Input: part model. Units: mm. Frame: model coordinates. Face numbers are marked on the shaded views. A direction names the side the tool comes from. Coordinates: 2 decimals unless noted, no trailing zeros. Order: outer loops, then holes, each group sorted by start corner. A loop starts at its lowest first (then second) coordinate and runs counter-clockwise, first axis right, second up. Notation, with made-up numbers: (41, -23) -> (54, -23) arc R22 cw to (54, 8) -> close; hole circle Ø3 at (85, 5). An arc over 180 degrees is marked (long way). Answer as CSV lines item,"result".
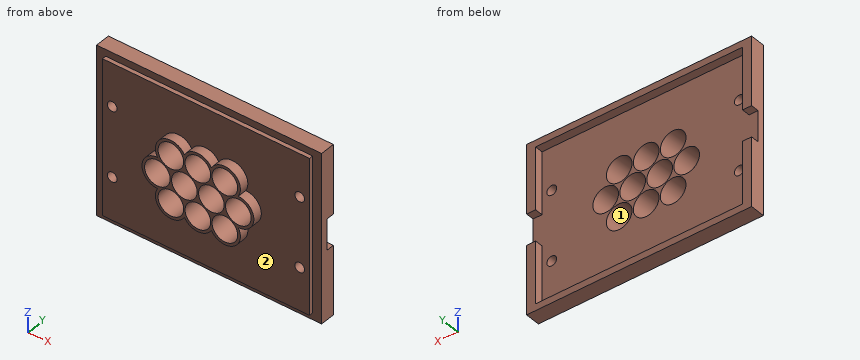
Autodesk Inventor part; units mm, degrees
ref_plane "YZ Plane" through (0, 0, 0) normal (1, 0, 0) x (0, 1, 0)
ref_plane "XZ Plane" through (0, 0, 0) normal (0, 1, 0) x (-1, 0, 0)
ref_plane "XY Plane" through (0, 0, 0) normal (0, 0, 1) x (1, 0, 0)
sketch "Sketch1" plane through (0, 0, 0) normal (0, 1, 0) x (-1, 0, 0)
  circle A0 centre (0, 0) radius 9.5
  circle A1 centre (20, 0) radius 9.5
  circle A2 centre (-20, 0) radius 9.5
  circle A3 centre (-10, 17.3205) radius 9.5
  circle A4 centre (10, 17.3205) radius 9.5
  circle A5 centre (30, 17.3205) radius 9.5
  circle A6 centre (10, -17.3205) radius 9.5
  circle A7 centre (30, -17.3205) radius 9.5
  circle A8 centre (-10, -17.3205) radius 9.5
  circle A9 centre (40, 0) radius 9.5
  line L0 (0, 0) -> (-32.9562, 0) construction
  line L1 (-32.9562, 0) -> (61.076, 0) construction
  circle A10 centre (0, 0) radius 10.5 construction
  circle A11 centre (-20, 0) radius 10.5 construction
  circle A12 centre (-10, -17.3205) radius 10.5 construction
  circle A13 centre (10, -17.3205) radius 10.5 construction
  circle A14 centre (30, -17.3205) radius 10.5 construction
  circle A15 centre (40, 0) radius 10.5 construction
  circle A16 centre (20, 0) radius 10.5 construction
  circle A17 centre (30, 17.3205) radius 10.5 construction
  circle A18 centre (10, 17.3205) radius 10.5 construction
  circle A19 centre (-10, 17.3205) radius 10.5 construction
  circle A20 centre (40, 0) radius 11.5 construction
  circle A21 centre (30, -17.3205) radius 11.5 construction
  circle A22 centre (10, -17.3205) radius 11.5 construction
  circle A23 centre (-10, -17.3205) radius 11.5 construction
  circle A24 centre (-20, 0) radius 11.5 construction
  circle A25 centre (-10, 17.3205) radius 11.5 construction
  circle A26 centre (10, 17.3205) radius 11.5 construction
  circle A27 centre (30, 17.3205) radius 11.5 construction
  circle A28 centre (0, 0) radius 11.5 construction
  circle A29 centre (20, 0) radius 11.5 construction
  arc A30 (39.9181, -11.4997) -> (39.9181, 11.4997) centre (39.9181, 0) ccw
  arc A31 (39.9181, 11.4997) -> (20, 22.9994) centre (30, 17.3205) ccw
  arc A32 (20, 22.9994) -> (0, 22.9994) centre (10, 17.3205) ccw
  arc A33 (0, 22.9994) -> (-19.9181, 11.4997) centre (-10, 17.3205) ccw
  arc A34 (-19.9181, 11.4997) -> (-19.9181, -11.4997) centre (-20, 0) ccw
  arc A35 (-19.9181, -11.4997) -> (0, -22.9994) centre (-10, -17.3205) ccw
  arc A36 (0, -22.9994) -> (20, -22.9994) centre (10, -17.3205) ccw
  arc A37 (20, -22.9994) -> (39.9181, -11.4997) centre (30, -17.3205) ccw
  point P0 (28.893, 7.4235)
  dimension "d0" = 19
  dimension "d2" = 19
  dimension "d4" = 19
  dimension "d6" = 19
  dimension "d8" = 19
  dimension "d10" = 19
  dimension "d11" = 19
  dimension "d13" = 19
  dimension "d14" = 19
  dimension "d53" = 19
  dimension "d91" = 1
  dimension "d144" = 21
  dimension "d145" = 21
  dimension "d146" = 21
  dimension "d147" = 21
  dimension "d148" = 21
  dimension "d149" = 21
  dimension "d150" = 21
  dimension "d151" = 21
  dimension "d152" = 21
  dimension "d153" = 21
  dimension "d154" = 23
  dimension "d155" = 23
  dimension "d156" = 23
  dimension "d157" = 23
  dimension "d158" = 23
  dimension "d159" = 23
  dimension "d160" = 23
  dimension "d161" = 23
  dimension "d162" = 23
  dimension "d163" = 23
extrude "Extrusion1" add sketch "Sketch1" along normal blind 15
sketch "Sketch4" plane through (0, 15, 0) normal (0, 1, 0) x (1, 0, 0)
  circle A0 centre (-30, 17.3205) radius 9.5
  circle A1 centre (-40, 0) radius 9.5
  circle A2 centre (-40, 0) radius 9.5
  circle A3 centre (10, 17.3205) radius 9.5
  circle A4 centre (-30, 17.3205) radius 9.5
  circle A5 centre (-10, 17.3205) radius 9.5
  circle A6 centre (-30, -17.3205) radius 9.5
  circle A7 centre (-10, -17.3205) radius 9.5
  circle A8 centre (10, -17.3205) radius 9.5
  circle A9 centre (20, 0) radius 9.5
  circle A10 centre (-20, 0) radius 9.5
  circle A11 centre (0, 0) radius 9.5
  line L0 (0, 0) -> (-9.528, 0) construction
  line L1 (-86.228, 57.7) -> (67.172, 57.7)
  line L2 (67.172, 57.7) -> (67.172, -57.7)
  line L3 (67.172, -57.7) -> (-86.228, -57.7)
  line L4 (-86.228, -57.7) -> (-86.228, 57.7)
  line L5 (-86.228, 57.7) -> (67.172, -57.7) construction
  line L6 (67.172, 57.7) -> (-86.228, -57.7) construction
  arc A12 (0, 22.9994) -> (-20, 22.9994) centre (-10, 17.3205) ccw
  arc A13 (19.9181, 11.4997) -> (0, 22.9994) centre (10, 17.3205) ccw
  arc A14 (19.9181, -11.4997) -> (19.9181, 11.4997) centre (20, 0) ccw
  arc A15 (0, -22.9994) -> (19.9181, -11.4997) centre (10, -17.3205) ccw
  arc A16 (-20, -22.9994) -> (0, -22.9994) centre (-10, -17.3205) ccw
  arc A17 (-39.9181, -11.4997) -> (-20, -22.9994) centre (-30, -17.3205) ccw
  circle A18 centre (-30, 17.3205) radius 11.5 construction
  arc A19 (-39.9181, 11.4997) -> (-39.9181, -11.4997) centre (-39.9181, 0) ccw
  arc A20 (-20, 22.9994) -> (-39.9181, 11.4997) centre (-30, 17.3205) ccw
  arc A21 (0, 22.9994) -> (-20, 22.9994) centre (-10, 17.3205) ccw
  arc A22 (19.9181, 11.4997) -> (0, 22.9994) centre (10, 17.3205) ccw
  arc A23 (19.9181, -11.4997) -> (19.9181, 11.4997) centre (20, 0) ccw
  arc A24 (0, -22.9994) -> (19.9181, -11.4997) centre (10, -17.3205) ccw
  arc A25 (-20, -22.9994) -> (0, -22.9994) centre (-10, -17.3205) ccw
  arc A26 (-39.9181, -11.4997) -> (-20, -22.9994) centre (-30, -17.3205) ccw
  arc A27 (-39.9181, 11.4997) -> (-39.9181, -11.4997) centre (-39.9181, 0) ccw
  arc A28 (-20, 22.9994) -> (-39.9181, 11.4997) centre (-30, 17.3205) ccw
  point P0 (-17.0502, -21.4927)
  point P1 (-17.0502, -11.5134)
  point P2 (-17.0502, -8.8009)
  point P3 (-17.0502, 8.8009)
  point P4 (-17.0502, 11.5134)
  point P5 (-17.0502, 21.4927)
  point P6 (-2.0059, 21.4927)
  point P7 (-2.0059, -11.5134)
  point P8 (-2.0059, -8.8009)
  point P9 (-2.0059, 8.8009)
  point P10 (-2.0059, 11.5134)
  point P11 (-2.0059, -21.4927)
  dimension "d104" = 153.4
  dimension "d164" = 115.4
extrude "Extrusion7" add sketch "Sketch4" against normal blind 8 contours L1 L2 L3 L4
sketch "Sketch5" plane through (0, 15, 0) normal (0, 1, 0) x (1, 0, 0)
  line L0 (-86.228, -57.7) -> (67.172, -57.7)
  line L1 (67.172, -57.7) -> (67.172, 57.7)
  line L2 (67.172, 57.7) -> (-86.228, 57.7)
  line L3 (-86.228, 57.7) -> (-86.228, -57.7)
  circle A0 centre (-40, 0) radius 9.5
  circle A1 centre (10, 17.3205) radius 9.5
  circle A2 centre (-30, 17.3205) radius 9.5
  circle A3 centre (-10, 17.3205) radius 9.5
  circle A4 centre (-30, -17.3205) radius 9.5
  circle A5 centre (-10, -17.3205) radius 9.5
  circle A6 centre (10, -17.3205) radius 9.5
  circle A7 centre (20, 0) radius 9.5
  circle A8 centre (-20, 0) radius 9.5
  circle A9 centre (0, 0) radius 9.5
  line L4 (-86.228, 57.7) -> (67.172, 57.7)
  line L5 (67.172, 57.7) -> (67.172, -57.7)
  line L6 (67.172, -57.7) -> (-86.228, -57.7)
  line L7 (-86.228, -57.7) -> (-86.228, 57.7)
  line L8 (-92.8745, -62.7) -> (73.8184, -62.7)
  line L9 (73.8184, -62.7) -> (73.8184, 62.7)
  line L10 (73.8184, 62.7) -> (-92.8745, 62.7)
  line L11 (-92.8745, 62.7) -> (-92.8745, -62.7)
  line L12 (-92.8745, -62.7) -> (73.8184, 62.7) construction
  line L13 (73.8184, -62.7) -> (-92.8745, 62.7) construction
  point P0 (66.922, -57.45)
  point P1 (-9.528, 0)
  dimension "d169" = 5
  dimension "d170" = 6.6464
  dimension "d171" = 166.6929
  dimension "d172" = 125.4
extrude "Extrusion8" add sketch "Sketch5" along normal blind 6 and the other way blind 5 contours L11 L10 L9 L8
sketch "Sketch6" plane through (0, 15, 0) normal (0, 1, 0) x (1, 0, 0)
  line L0 (59.944, 57.1514) -> (59.944, 25.95) construction
  line L1 (59.944, 25.95) -> (67.172, 25.95) construction
  line L2 (-79, -57.7) -> (-79, -25.95) construction
  line L3 (-79, -25.95) -> (-86.228, -25.95) construction
  circle A0 centre (59.944, 25.95) radius 3.615
  circle A1 centre (59.944, -25.95) radius 3.615
  circle A2 centre (-79, -25.95) radius 3.615
  circle A3 centre (-79, 25.95) radius 3.615
  line L4 (73.8184, -62.7) -> (73.8184, 62.7)
  line L5 (73.8184, 62.7) -> (-92.8745, 62.7)
  line L6 (-92.8745, 62.7) -> (-92.8745, -62.7)
  line L7 (-92.8745, -62.7) -> (73.8184, -62.7)
  line L8 (-86.228, -57.7) -> (-86.228, 57.7)
  line L9 (-86.228, 57.7) -> (67.172, 57.7)
  line L10 (67.172, 57.7) -> (67.172, -57.7)
  line L11 (67.172, -57.7) -> (-86.228, -57.7)
  line L12 (-86.228, -57.7) -> (67.172, -57.7)
  line L13 (67.172, -57.7) -> (67.172, 57.7)
  line L14 (67.172, 57.7) -> (-86.228, 57.7)
  line L15 (-86.228, 57.7) -> (-86.228, -57.7)
  circle A4 centre (-40, 0) radius 9.5
  circle A5 centre (10, 17.3205) radius 9.5
  circle A6 centre (-30, 17.3205) radius 9.5
  circle A7 centre (-10, 17.3205) radius 9.5
  circle A8 centre (-30, -17.3205) radius 9.5
  circle A9 centre (-10, -17.3205) radius 9.5
  circle A10 centre (10, -17.3205) radius 9.5
  circle A11 centre (20, 0) radius 9.5
  circle A12 centre (-20, 0) radius 9.5
  circle A13 centre (0, 0) radius 9.5
  line L16 (-86.228, 57.7) -> (67.172, 57.7)
  line L17 (67.172, 57.7) -> (67.172, -57.7)
  line L18 (67.172, -57.7) -> (-86.228, -57.7)
  line L19 (-86.228, -57.7) -> (-86.228, 57.7)
  dimension "d123" = 7.23
  dimension "d124" = 7.23
  dimension "d125" = 7.23
  dimension "d140" = 7.23
  dimension "d179" = 31.75
  dimension "d180" = 7.228
  dimension "d181" = 7.228
  dimension "d182" = 31.75
  dimension "d183" = 31.75
  dimension "d184" = 7.228
  dimension "d185" = 7.228
  dimension "d186" = 31.75
extrude "Extrusion6" cut sketch "Sketch6" against normal through all contours A0 | A1 | A2 | A3
sketch "Sketch7" plane through (-92.8745, 10, 62.7) normal (-1, 0, 0) x (0, 0, 1)
  line L0 (-74.1997, -10) -> (-74.1997, -3)
  line L1 (-51.2003, -10) -> (-51.2003, -3)
  line L2 (-120.4, 5) -> (-5, 5)
  line L3 (0, 0) -> (-125.4, 0)
  line L4 (-125.4, 11) -> (0, 11)
  line L5 (-74.1997, 5) -> (-51.2003, 5)
  line L6 (-51.2003, 5) -> (-51.2003, 11)
  line L7 (-51.2003, 11) -> (-74.1997, 11)
  line L8 (-74.1997, 11) -> (-74.1997, 5)
  point P0 (-62.7, -10)
extrude "Extrusion9" cut sketch "Sketch7" against normal through all
properties part number "BatteryCasev1_3DPrint"
1. Cut plane C-C (z = -35). Return the cut outline in (x, y).
Findings:
outline,"(-92.87, 10) -> (-86.23, 10) -> (-86.23, 7) -> (67.17, 7) -> (67.17, 10) -> (73.82, 10) -> (73.82, 21) -> (67.17, 21) -> (67.17, 15) -> (-86.23, 15) -> (-86.23, 21) -> (-92.87, 21) -> close"
2. Cut plane B-B (y = 18.25). Return the cut outline in (x, z).
Findings:
outline,"(-92.87, -62.7) -> (73.82, -62.7) -> (73.82, -11.5) -> (67.17, -11.5) -> (67.17, -57.7) -> (-86.23, -57.7) -> (-86.23, -11.5) -> (-92.87, -11.5) -> close; (-92.87, 11.5) -> (-86.23, 11.5) -> (-86.23, 57.7) -> (67.17, 57.7) -> (67.17, 11.5) -> (73.82, 11.5) -> (73.82, 62.7) -> (-92.87, 62.7) -> close"
3. Cut plane A-A (x = -79). Return the cut outline in (y, z) (3 decimals).
Findings:
outline,"(7, -57.7) -> (10, -57.7) -> (10, -62.7) -> (21, -62.7) -> (21, -57.7) -> (15, -57.7) -> (15, -29.565) -> (7, -29.565) -> close; (7, -22.335) -> (15, -22.335) -> (15, 22.335) -> (7, 22.335) -> close; (7, 29.565) -> (15, 29.565) -> (15, 57.7) -> (21, 57.7) -> (21, 62.7) -> (10, 62.7) -> (10, 57.7) -> (7, 57.7) -> close"
4. Cut plane D-D (x = 39). Return the cut outline in (y, z), plus the area to 3 significant figures.
Findings:
outline,"(7, -57.7) -> (10, -57.7) -> (10, -62.7) -> (21, -62.7) -> (21, -57.7) -> (15, -57.7) -> (15, 57.7) -> (21, 57.7) -> (21, 62.7) -> (10, 62.7) -> (10, 57.7) -> (7, 57.7) -> close"
area,"1,030 mm2"
5. Ray query, line 1 along Z through (x, y) = (-79, 9.75) (3 decimals); line 2 along Z through (x, y) = (-79, 13) (3 decimals); line 3 along X through (y, z) = (18.25, 54.5). Return the intervals inside material, ascending.
Findings:
line 1,"z = -57.7 to -29.565, -22.335 to 22.335, 29.565 to 57.7"
line 2,"z = -62.7 to -29.565, -22.335 to 22.335, 29.565 to 62.7"
line 3,"x = -92.87 to -86.23, 67.17 to 73.82"
6. Contact query for flat-ended pins moving along their axis: pin 1 (3 mm diameter, centred on x = 33, z = -14, fed in from +Y); pin 2 (1.5 mm diameter, centred on x = 23, y = 9, fed in from +Z); pin 3 (1.5 mm diameter, centred on y = 7.5, z = 15, fed in from -X); pin 4 (17 mm diameter, centred on x = 20, z = 0, fed in from -Y). Output: stop coordinate, or through.
Findings:
pin 1,"stops at y = 15"
pin 2,"stops at z = 57.7"
pin 3,"stops at x = -86.23"
pin 4,"passes through"
7. Reachability of the marked faces 1 and 2 from +Z, -Z, +X, -X, +Y, -Y: full face, straight path, thin tool, end or side. Return the list, or none.
Findings:
face 1,"+Y, -Y"
face 2,"-Y"
